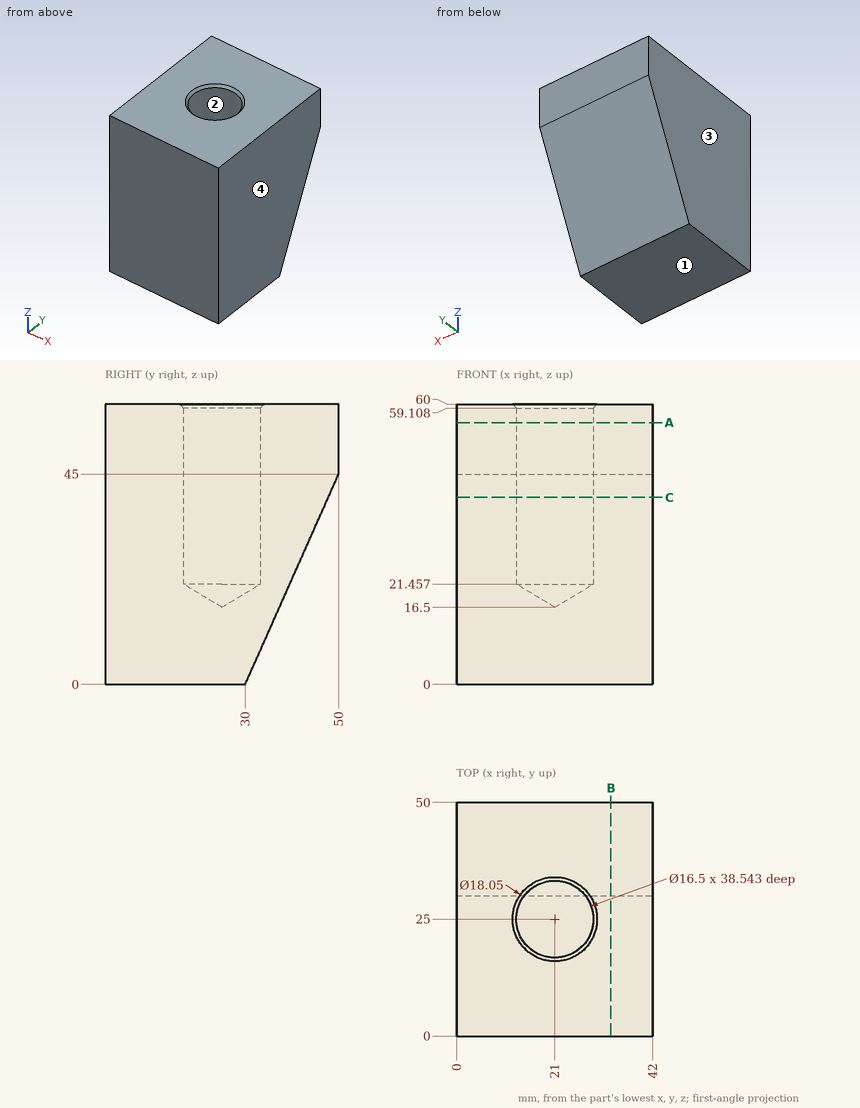
The figure shows three views and two pictorial views of one solid part (mm, origin at its lowest corner). Answer the questions. Round coordinates to 2 decimals unless told otherwise and drop trailing zeros. Order: outer loops, then holes, each group sorted by start corner. A loop starts at its lowest first (then second) coordinate and runs counter-clockwise, first axis right, second up. Notation, with made-up numbers: M 47.5,5.5 L 90.5,5.5 A22 cw 90.5,33.5 Z; hole C 45,-10.5 d1. An arc over 180 degrees is marked long. Answer in a Markdown table with one row per item. Add a question column.
1) The part is cut by section B-B on x = 33. Determine the outline of the cut face in (y, z).
2) Flat-ended cylindrical pins translate along their axes: pin 1 Ø6 at (x, y) = (10.5, 40) entering from -Z; pin 2 Ø3 at (x, z) = (9.5, 18) entering from +Y; pin 3 Ø1 at (x, z) = (13, 35.5) entering from +Y; pin 4 Ø6 at (y, z) = (38.5, 8.5) entering from +X. Find the tip coordinate at first contact, or state that the pin passes through.
3) Consider line 1 along X through (y, z) = (25, 39.5); line 2 along Y through (x, z) = (27.5, 38); line 3 along Y through (x, z) = (23, 28) (1 decimal). Determine where each line is inside the solid, lowest interval first. Write a range as from..to.
4) The part is cut by section A-A on z = 56. Determine the outline of the cut face in (x, y).
5) Determine the mould class of the marked faces 1, 2, 3 and 4 for opening direction X: pulls with the +X half, pulls with the -X half, needs draft (parallel to the pull), parting line crosses it, or undercut.
6) The part is cut by section C-C on z = 40. Determine the outline of the cut face in (x, y).
Findings below:
| question | item | result |
|---|---|---|
| 1 | outline | M 0,0 L 30,0 L 50,45 L 50,60 L 0,60 Z |
| 2 | pin 1 | stops at z = 15.75 |
| 2 | pin 2 | stops at y = 38.67 |
| 2 | pin 3 | stops at y = 46 |
| 2 | pin 4 | passes through |
| 3 | line 1 | x = 0..12.75, 29.25..42 |
| 3 | line 2 | y = 0..19.92, 30.08..46.89 |
| 3 | line 3 | y = 0..17, 33..42.4 |
| 4 | outline | M 0,0 L 42,0 L 42,50 L 0,50 Z; hole C 21,25 d16.5 |
| 5 | face 1 | needs draft |
| 5 | face 2 | undercut |
| 5 | face 3 | pulls with the -X half |
| 5 | face 4 | pulls with the +X half |
| 6 | outline | M 0,0 L 42,0 L 42,47.78 L 0,47.78 Z; hole C 21,25 d16.5 |
